```python
from build123d import *

# Parameters (mm, degrees)
SKETCH1_W           = 20
SKETCH1_H           = 6
BOSS_EXTRUDE1_DEPTH = 13
SKETCH2_R           = 1.5
BOSS_EXTRUDE3_DEPTH = 34
SKETCH6_R           = 3.50549755
BOSS_EXTRUDE4_DEPTH = 5


with BuildPart() as part:
    # Sketch1 → Boss-Extrude1 (new body)
    with BuildSketch(Plane(origin=(0, 0, 0), x_dir=(1, 0, 0), z_dir=(0, 1, 0))):
        with Locations((10, 3)):
            Rectangle(SKETCH1_W, SKETCH1_H)
    extrude(amount=BOSS_EXTRUDE1_DEPTH)

    # Sketch2 → Boss-Extrude3 (add)
    with BuildSketch(Plane.XZ):
        with Locations(Location((10, -3, 0), (0, 0, 270))):
            Circle(SKETCH2_R)
    extrude(amount=-BOSS_EXTRUDE3_DEPTH)

    # Sketch5 → Revolve1 (revolve)
    with BuildSketch(Plane.XY.offset(-3), mode=Mode.PRIVATE) as revolve1_sk:
        with BuildLine():
            Line((10, 34), (10, 26.687164187))
            Line((10, 26.687164187), (-2.865987709, 26.687164187))
            add(Edge.make_bspline(
                [(10, 34), (2.373080753, 34.40580884), (-2.865987709, 26.687164187)],
                knots=[0, 0, 0, 1, 1, 1], degree=2))
        make_face()
    revolve(revolve1_sk.sketch.rotate(Axis((10, 34, -3), (0, -1, 0)), 90), axis=Axis((10, 34, -3), (0, -1, 0)))

    # Sketch6 → Boss-Extrude4 (add)
    with BuildSketch(Plane(origin=(0, 0, -6), x_dir=(-1, 0, 0), z_dir=(0, 0, -1))):
        with Locations(Location((-6.235505229, 6.359969697, 0), (0, 0, 180))):
            Circle(SKETCH6_R)
    extrude(amount=BOSS_EXTRUDE4_DEPTH)


solid = part.part
```
Design review of the part built by this model. Coordinates are the model's own, in mm. A direction names the side the tool comes from. Give positions to 0.01 mm unless a question says otherwise; leave off trailing zeros. Order: outer loops, then holes, each group sorted by start corner. A loop starts at its lowest first (then second) coordinate and runs counter-clockwise, first axis right, second up. Notation, with made-up numbers: (71, 84.25) -> (80, 84.25) arc R19 cw to (80, 93.25) -> close; hole circle Ø4 at (72.5, -7). An arc over 180 degrees is marked (long way). Write item = value, one per line. Start each with the question number.
(1) For faces 1 (the face through (3.45, 8.49, -8.46)), 2 (the face through (0, 6, -3)), 3 (the face through (20, 6, -3)), list the 3-axis set-ups (+Z, -Z, +X, -X, +Y, -Y) from which the entire face can be reached by the end or side of a thin tool; tool diameter is ignored.
(2) We need section A-A on y = 12. Write out the cut boundary in (x, z).
(3) To check wall thickness, follow line 1 along Y through (x, z) = (2.25, -4); line 2 along Y through (x, z) = (6.5, -8.75); line 3 along Z through (x, y) = (2.5, 8.5). State the ranges of each line that lie inside material, in increasing order.
(4) For pin 1 (1.8 mm diameter, centred on x = 14, z = -2.5, fed in from +Y); pin 2 (1 mm diameter, centred on x = 11, z = -7, fed in from -Y); pin 3 (6 mm diameter, centred on x = 2.5, y = 12, fed in from -Z); pin 4 (12 mm diameter, centred on x = 13, y = 26, fed in from +Z), all flat-tipped, find the tip position at first contact; note any pin that passes through.
Numbers:
q1.face_1 = -Z
q1.face_2 = +Z, -Z, -X, -Y
q1.face_3 = +Z, -Z, +X, -Y
q2.outline = (0, -6) -> (20, -6) -> (20, 0) -> (0, 0) -> close
q3.line_1 = 0 to 13, 26.69 to 31.89
q3.line_2 = 2.86 to 9.86, 26.69 to 32.54
q3.line_3 = -6 to 0
q4.pin_1 = 33.81
q4.pin_2 = 26.69
q4.pin_3 = -6
q4.pin_4 = 9.87
